Read the model definition and answer for the solid it produces. Units are mm, in the model's axes. A direction names the side the tool comes from. Round coordinates to 2 decimals unless told otherwise and drop trailing zeros. Order: outer loops, then holes, each group sorted by start corner. A loop starts at its lowest first (then second) coordinate and runs counter-clockwise, first axis right, second up.
from build123d import *

# Parameters (mm, degrees)
F1_DEPTH  = 2
F2_W      = 17
F2_H      = 24
F3_DEPTH  = 1
F4_W      = 12
F4_H      = 15
F5_DEPTH  = 2.5
F6_W      = 8
F6_H      = 6
F7_DEPTH  = 3
F8_W      = 2
F8_H      = 4.5
F9_DEPTH  = 2
F10_W     = 2
F10_H     = 1
F11_DEPTH = 1
F12_W     = 10.5
F12_H     = 4
F13_DEPTH = 1.5
F14_R     = 0.375
F15_DEPTH = 25
F16_R     = 4
F17_R     = 1


with BuildPart() as f1:
    # F0 (on Top) → F1 (new body)
    with BuildSketch(Plane.XY):
        Polygon((13, 17), (-13, 17), (-13, -11), (-10, -11), (-10, -17), (13, -17), align=None)
    extrude(amount=F1_DEPTH)

    # F2 (on face) → F3 (join)
    with BuildSketch(Plane.XY.offset(2)):
        with Locations((0, 5)):
            Rectangle(F2_W, F2_H)
    extrude(amount=F3_DEPTH)

    # F4 (on face) → F5 (join)
    with BuildSketch(Plane.XY.offset(3)):
        with Locations((0, 1.5)):
            Rectangle(F4_W, F4_H)
    extrude(amount=F5_DEPTH)

    # F6 (on face) → F7 (join)
    with BuildSketch(Plane(origin=(0, 0, 0), x_dir=(1, 0, 0), z_dir=(0, 0, -1))):
        with Locations((0, 14)):
            Rectangle(F6_W, F6_H)
    extrude(amount=F7_DEPTH)

    # F8 (on face) → F9 (join)
    with BuildSketch(Plane(origin=(0, 0, 0), x_dir=(1, 0, 0), z_dir=(0, 0, -1))):
        with Locations((-9, 13.75)):
            Rectangle(F8_W, F8_H)
    extrude(amount=F9_DEPTH)

    # F10 (on face) → F11 (join)
    with BuildSketch(Plane(origin=(-10, 0, 0), x_dir=(0, -1, 0), z_dir=(-1, 0, 0))):
        with Locations((13.75, -1)):
            Rectangle(F10_W, F10_H)
    extrude(amount=F11_DEPTH)

    # F12 (on face) → F13 (join)
    with BuildSketch(Plane(origin=(0, 0, 0), x_dir=(1, 0, 0), z_dir=(0, 0, -1))):
        with Locations((-0.75, 0.206931)):
            Rectangle(F12_W, F12_H)
    extrude(amount=F13_DEPTH)

    # F14 (on face) → F15 (cut)
    with BuildSketch(Plane(origin=(0, 0, 0), x_dir=(1, 0, 0), z_dir=(0, 0, -1))):
        with Locations((-11.5, -9)):
            Circle(F14_R)
        with Locations((-11.5, -6.5)):
            Circle(F14_R)
        with Locations((-11.5, -4)):
            Circle(F14_R)
        with Locations((-11.5, -1.5)):
            Circle(F14_R)
        with Locations((-11.5, 1)):
            Circle(F14_R)
        with Locations((-11.5, 3.5)):
            Circle(F14_R)
        with Locations((-11.5, 6)):
            Circle(F14_R)
        with Locations((-11.5, 8.5)):
            Circle(F14_R)
        with Locations((11.5, -9)):
            Circle(F14_R)
        with Locations((11.5, -6.5)):
            Circle(F14_R)
        with Locations((11.5, -4)):
            Circle(F14_R)
        with Locations((11.5, -1.5)):
            Circle(F14_R)
        with Locations((11.5, 1)):
            Circle(F14_R)
        with Locations((11.5, 3.5)):
            Circle(F14_R)
        with Locations((11.5, 6)):
            Circle(F14_R)
        with Locations((11.5, 8.5)):
            Circle(F14_R)
    extrude(amount=-F15_DEPTH, mode=Mode.SUBTRACT)

    # F16
    f16_edges = [f1.edges().sort_by_distance(p)[0] for p in [
        (-13, 17, 1),
        (13, 17, 1),
    ]]
    fillet(f16_edges, radius=F16_R)

    # F17
    f17_edges = [f1.edges().sort_by_distance(p)[0] for p in [
        (-10, -17, 1),
        (13, -17, 1),
    ]]
    fillet(f17_edges, radius=F17_R)


solid = f1.part
Q1. A cutting plane is placed at B-B, the plane y = -1. Give the vertices of the cut face in (x, z) (3 decimals).
Outcome:
outline: (-13, 0) - (-11.875, 0) - (-11.875, 2) - (-13, 2) - close; (-11.125, 0) - (-6, 0) - (-6, -1.5) - (4.5, -1.5) - (4.5, 0) - (11.125, 0) - (11.125, 2) - (8.5, 2) - (8.5, 3) - (6, 3) - (6, 5.5) - (-6, 5.5) - (-6, 3) - (-8.5, 3) - (-8.5, 2) - (-11.125, 2) - close; (11.875, 0) - (13, 0) - (13, 2) - (11.875, 2) - close
Q2. A cutting plane is placed at A-A, the plane z = 0.75. Give the number of separate pieces and of enclosed holes in the cut face, plus the area to 3 significant figures.
Outcome:
separate pieces: 1
enclosed holes: 16
area: 852 mm2
Q3. A cutting plane is placed at C-C, the plane x = 5.5. Give the vertices of the cut face in (y, z), plus the area to 4 significant figures.
Outcome:
outline: (-17, 0) - (17, 0) - (17, 3) - (9, 3) - (9, 5.5) - (-6, 5.5) - (-6, 3) - (-7, 3) - (-7, 2) - (-17, 2) - close
area: 129.5 mm2
Q4. Flat-ended cylindrical pins translate along their axes: pin 1 (2 mm diameter, centred on x = 1, y = 0.5, fed in from -Z); pin 2 (2 mm diameter, centred on x = -9, y = -14.5, fed in from -Z); pin 3 (0.6 mm diameter, centred on x = -9, z = -1, fed in from +Y). Find the tip coordinate at first contact, or state that the pin passes through.
Outcome:
pin 1: stops at z = -1.5
pin 2: stops at z = -2
pin 3: stops at y = -11.5
Q5. Straight lines are drawn through the part: probe 1 along X at (y, z) = (-3.5, 1.2) (3 decimals); probe 2 along Y at (x, z) = (2.5, -1); probe 3 along Y at (x, z) = (-10.5, -1). For each, find the intervals that lie inside material, in ascending order.
Outcome:
probe 1: x = -13 to -11.875, -11.125 to 11.125, 11.875 to 13
probe 2: y = -17 to -11, -2.21 to 1.79
probe 3: y = -14.75 to -12.75
Q6. For faces 1 (the face through (0, 9, 4)), 2 (the face through (-12, -11, 1)), 3 (the face through (-0.1, -7, 2.5)), determine the directions among +Z, -Z, +X, -X, +Y, -Y from which every point of the face is accessible in a straight line to the end or side of a thin tool.
Outcome:
face 1: +Z, +X, -X, +Y
face 2: +Z, -Z, -X, -Y
face 3: +Z, +X, -X, -Y
Q7. A cutting plane is placed at D-D, the plane y = 4. Give the vertices of the cut face in (x, z) (3 decimals), plus the area to 3 significant figures.
Outcome:
outline: (-13, 0) - (-11.875, 0) - (-11.875, 2) - (-13, 2) - close; (-11.125, 0) - (11.125, 0) - (11.125, 2) - (8.5, 2) - (8.5, 3) - (6, 3) - (6, 5.5) - (-6, 5.5) - (-6, 3) - (-8.5, 3) - (-8.5, 2) - (-11.125, 2) - close; (11.875, 0) - (13, 0) - (13, 2) - (11.875, 2) - close
area: 96.0 mm2
Q8. For a pull along X with two mould halves and no side action, classify faces 4 (the face through (-1, 1.793, -1)), 5 (the face through (-8, -14, -1)), 6 (the face through (-11, -14, -1)) as released by +X, released by -X, zero draft, split by the parting line, or undercut.
Outcome:
face 4: zero draft
face 5: undercut
face 6: released by -X
